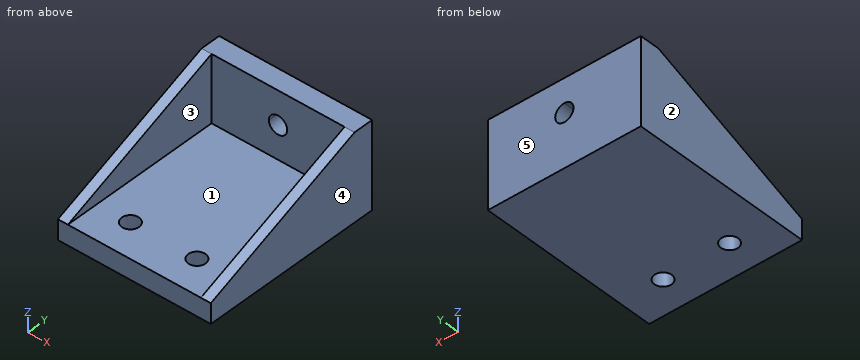
```python
from build123d import *

# Parameters (mm, degrees)
F0_W     = 40
F0_H     = 20
F0_R     = 2.6
F0_H_2   = 29
F1_DEPTH = 6
F0_H_3   = 6
F2_DEPTH = 26
F4_DEPTH = 3
F6_DEPTH = 25


# Not quite as in the source:
# - a pattern or mirror of a feature is missing from the dataset's text; its kind, count and spacing are read off the source's solid


with BuildPart() as f1:
    # F0 (on Top) → F1 (new body)
    with BuildSketch(Plane.XY):
        Rectangle(F0_W, F0_H)
        with Locations((-10, 0)):
            Circle(F0_R, mode=Mode.SUBTRACT)
        with Locations((10, 0)):
            Circle(F0_R, mode=Mode.SUBTRACT)
        with Locations((0, 24.5)):
            Rectangle(F0_W, F0_H_2)
    extrude(amount=F1_DEPTH)

    # F0 (on Top) → F2 (join)
    with BuildSketch(Plane.XY):
        with Locations((0, 42)):
            Rectangle(F0_W, F0_H_3)
    extrude(amount=F2_DEPTH)

    # F3 (on face) → F4 (join)
    with BuildSketch(Plane(origin=(-20, 0, 0), x_dir=(0, -1, 0), z_dir=(-1, 0, 0))):
        Polygon((10, 0), (10, 6), (-39, 26), (-45, 26), (-45, 0), align=None)
    f4 = extrude(amount=F4_DEPTH)

    # F4_copies: F4 across plane
    add(f4.mirror(Plane(origin=(0, 0, 0), x_dir=(0, 0, 1), z_dir=(1, 0, 0))))

    # F5 (on face) → F6 (cut)
    with BuildSketch(Plane(origin=(0, 45, 0), x_dir=(-1, 0, 0), z_dir=(0, 1, 0))):
        with BuildLine():
            ThreePointArc((0, 18.75), (-1.9445436483, 14.0554563517), (2.75, 16))
            ThreePointArc((2.75, 16), (1.9445436483, 17.9445436483), (0, 18.75))
        make_face()
    extrude(amount=-F6_DEPTH, mode=Mode.SUBTRACT)


solid = f1.part
```
Input: part model. Units: mm. Frame: model coordinates. Face numbers are marked on the shaded views. A direction names the side the tool comes from. Round coordinates to 2 decimals unless told otherwise and drop trailing zeros. Loops run counter-clockwise (first coordinate to the right, second up) from the corner with the lowest first, then second, coordinate; pieces in that order, holes last. Notation, with made-up numbers: (-38, 62) - (-17, 62) arc R25 ccw to (-17, 94) - close; hole circle Ø2 at (27, 2.25). An arc over 180 degrees is marked (long way). One line per item, written item: value. Start each with the question number.
(1) Section C-C, the plane z = 15.25. Return loops of the section in (x, y).
(2) Ray query, line 1 (X direction, y = 41.85, z = 16); line 2 (Z direction, x = 0, y = 43.05); line 3 (Y direction, x = 10, z = 1.9). Return the intervals inside material, ascending. Write a range as [from, to].
(3) Section B-B, the plane z = 2.75. Return loops of the section in (x, y).
(4) Draft query along X for the marked faces 3, 4 and 5. Return one class per face: +X half, -X half, draft (parallel to the pull), parting line (faces both ways), or undercut.
(5) Section A-A, the plane x = 10. Return loops of the section in (y, z), plus the area to 3 significant figures.
(6) Section D-D, the plane y = 0. Return loops of the section in (x, z).
(7) Access query for the marked faces 1 and 2. Directions: +Z, -Z, +X, -X, +Y, -Y. A direction counts if a zero-diameter tool reaches every point of the face in a straight line with its end or side. Return the directions, or none.
(8) Contact query for flat-ended pins moving along their axis: P1, Ø20, axis at x = 4, y = 14.5, coming from the +Z side; P2, Ø3, axis at x = 8, z = 9, coming from the -Y side. Output: stop coordinate, or through.
Results below:
1. outline: (-23, 12.66) - (-20, 12.66) - (-20, 39) - (-2.65, 39) - (-2.65, 45) - (-23, 45) - close; (2.65, 39) - (20, 39) - (20, 12.66) - (23, 12.66) - (23, 45) - (2.65, 45) - close
2. line 1: [-23, -2.75], [2.75, 23]
2. line 2: [0, 13.25], [18.75, 26]
2. line 3: [-10, -2.6], [2.6, 45]
3. outline: (-23, -10) - (23, -10) - (23, 45) - (-23, 45) - close; hole circle Ø5.2 at (-10, 0); hole circle Ø5.2 at (10, 0)
4. face 3: undercut
4. face 4: +X half
4. face 5: draft
5. outline: (-10, 0) - (-2.6, 0) - (-2.6, 6) - (-10, 6) - close; (2.6, 0) - (45, 0) - (45, 26) - (39, 26) - (39, 6) - (2.6, 6) - close
5. area: 419 mm^2
6. outline: (-23, 0) - (-12.6, 0) - (-12.6, 6) - (-20, 6) - (-20, 10.08) - (-23, 10.08) - close; (-7.4, 0) - (7.4, 0) - (7.4, 6) - (-7.4, 6) - close; (12.6, 0) - (23, 0) - (23, 10.08) - (20, 10.08) - (20, 6) - (12.6, 6) - close
7. face 1: +Z, -Y
7. face 2: +Z, -Z, -X, +Y, -Y
8. P1: z = 6
8. P2: y = 39
